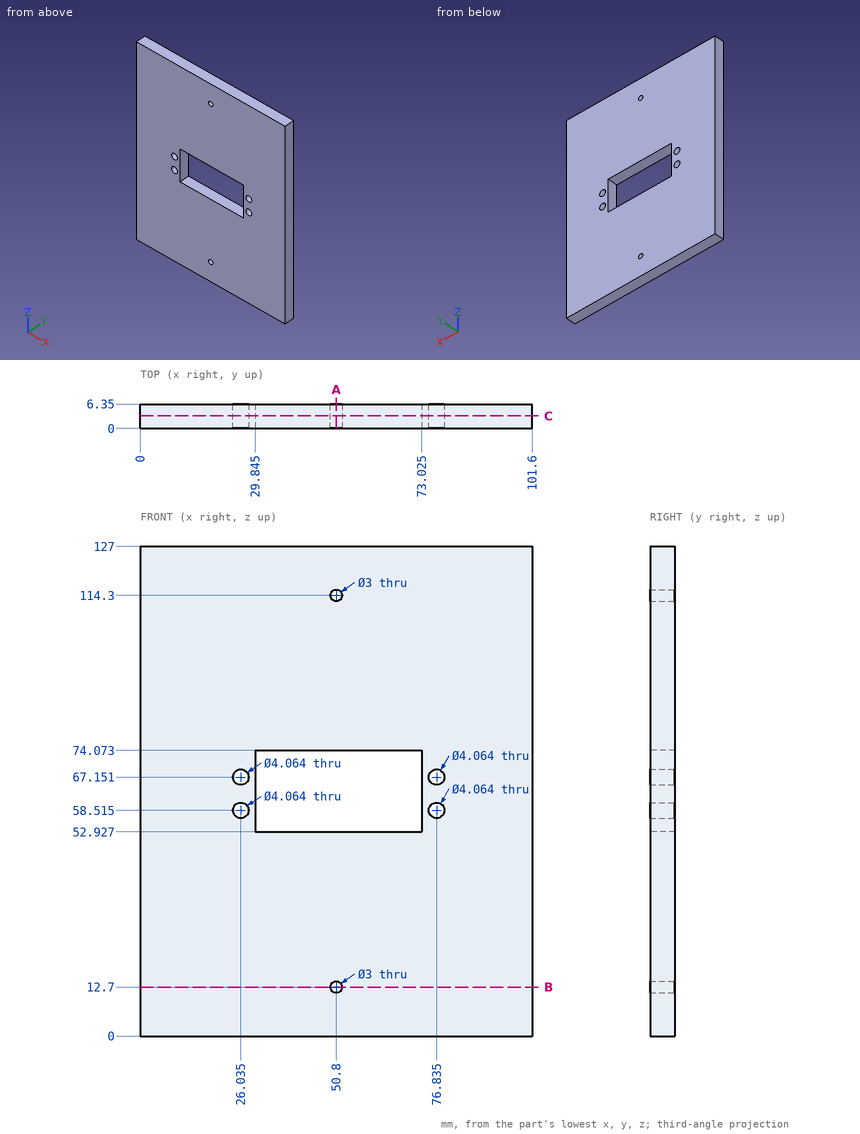
Here's the drawing with two shaded views (mm, measured from the low corner). I have some questions. Coordinates: 2 decimals unless noted, no trailing zeros. Loops run counter-clockwise (first coordinate to the right, second up) from the corner with the lowest first, then second, coordinate; pieces in that order, holes last. Notation, with made-up numbers: (-21.5, 38.5) -> (-9.5, 38.5) arc R12 ccw to (-9.5, 45.5) -> close; hole circle Ø2 at (50.5, -20). An arc over 180 degrees is marked (long way). Answer as a JSON object with one key per item and string values.
1) For P1, Ø3.5, axis at x = 76.83, z = 67.15, coming from the -Y side, with a flat end and sliding along its axis, tell me the tip position at first contact or that it passes through.
Results:
{"P1": "passes through"}
2) Imagine slicing it at B-B (z = 12.7). Please give me the cut outline in (x, y), then the cut area to 3 significant figures.
Results:
{"outline": "(0, 0) -> (49.3, 0) -> (49.3, 6.35) -> (0, 6.35) -> close; (52.3, 0) -> (101.6, 0) -> (101.6, 6.35) -> (52.3, 6.35) -> close", "area": "626 mm^2"}
3) Imagine slicing it at A-A (x = 50.8). Please give me the cut outline in (y, z).
Results:
{"outline": "(0, 0) -> (6.35, 0) -> (6.35, 11.2) -> (0, 11.2) -> close; (0, 14.2) -> (6.35, 14.2) -> (6.35, 52.93) -> (0, 52.93) -> close; (0, 74.07) -> (6.35, 74.07) -> (6.35, 112.8) -> (0, 112.8) -> close; (0, 115.8) -> (6.35, 115.8) -> (6.35, 127) -> (0, 127) -> close"}
4) If I drill on line 1 (X direction, y = 5, z = 12.5); line 2 (Z direction, x = 50.8, y = 3.5); line 3 (Z direction, x = 43.5, y = 5.5), over which ranges is the centre line in solid material (lowest first)?
Results:
{"line 1": "x = 0 to 49.31, 52.29 to 101.6", "line 2": "z = 0 to 11.2, 14.2 to 52.93, 74.07 to 112.8, 115.8 to 127", "line 3": "z = 0 to 52.93, 74.07 to 127"}
5) Imagine slicing it at C-C (y = 3.25). Please give me the cut outline in (x, z) (1 decimal).
Results:
{"outline": "(0, 0) -> (101.6, 0) -> (101.6, 127) -> (0, 127) -> close; hole circle Ø4.1 at (26, 58.5); hole circle Ø4.1 at (26, 67.2); hole (29.8, 52.9) -> (73, 52.9) -> (73, 74.1) -> (29.8, 74.1) -> close; hole circle Ø3 at (50.8, 12.7); hole circle Ø3 at (50.8, 114.3); hole circle Ø4.1 at (76.8, 58.5); hole circle Ø4.1 at (76.8, 67.2)"}
